Answer from the drawing. Dimensions are ordinates in mm from the lowest x, y and z of the part. A direction names the side the tool comes from. Give positions to 0.01 mm unless a question says otherwise; leave off trailing zeros. Loops run counter-clockwise (first coordinate to the right, second up) from the corner with the lowest first, then second, coordinate; pieces in that order, holes last. Notation, with made-up numbers: (-18, 21) -> (37, 21) arc R24 ccw to (37, 31) -> close; hole circle Ø3 at (-16.75, -31). An arc over 180 degrees is marked (long way). Return JSON: item names as keys, results as strings. Group by question number.
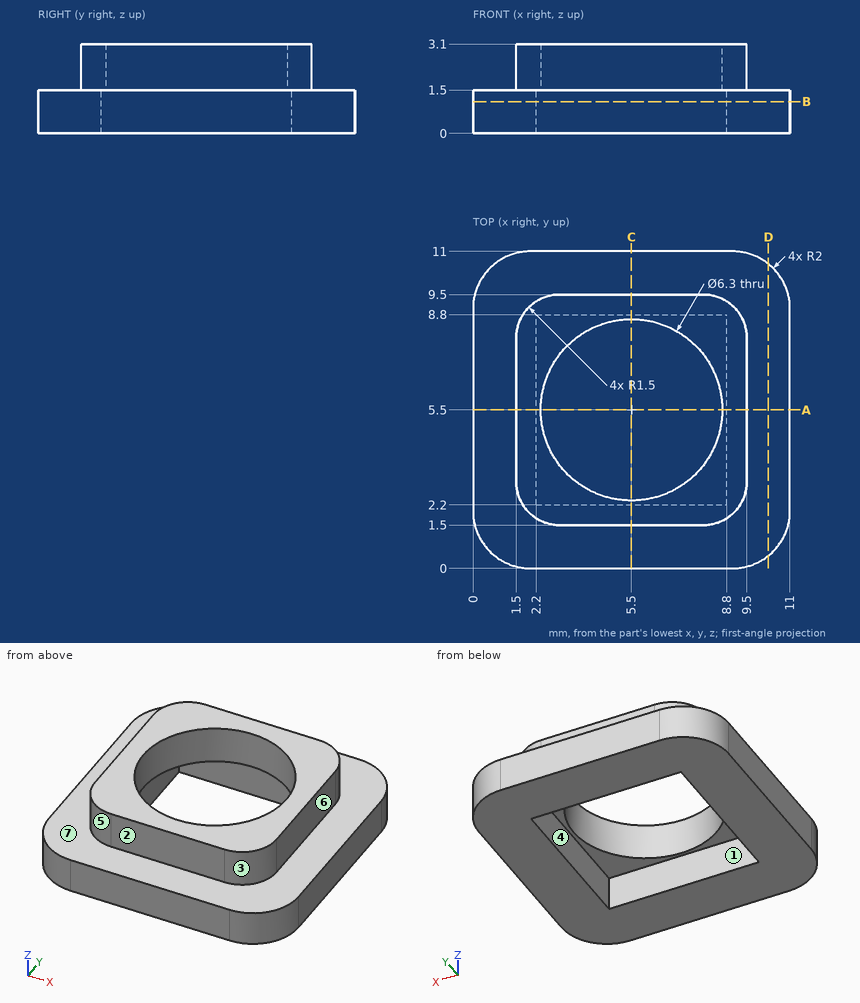
1. Straight lines are drawn through the part: line 1 (Y direction, x = 5.5, z = 2); line 2 (Y direction, x = 6, z = 1). For each, find the intervals that lie inside material, in ascending order. Write a range as from..to.
2. Section A-A on y = 5.5 is taken. Determine the outline of the cut face in (x, z).
3. Section D-D on x = 10.25 is taken. Determine the outline of the cut face in (y, z).
4. Section B-B on z = 1.1 is taken. Determine the outline of the cut face in (x, y), then the cut area to 3 significant figures.
5. Which of the six approach directions +Z, -Z, +X, -X, +Y, -Y give full straight-line access (tool end or side, diameter ignored) to the marked faces 4, 5, 6 and 7?
6. Flat-ended cylindrical pins translate along their axes: pin 1 Ø0.8 at (y, z) = (6, 2.5) entering from +X; pin 2 Ø1.3 at (y, z) = (5.5, 2.5) entering from -X; pin 3 Ø1.3 at (x, z) = (5.5, 2.5) entering from -Y. Find the tip coordinate at first contact, or state that the pin passes through.
7. Determine the mould class of the marked faces 1, 2 and 3 for opening direction X: pulls with the +X half, pulls with the -X half, needs draft (parallel to the pull), parting line crosses it, or undercut.
Completed:
{
 "1": {"line 1": "y = 1.5..2.35, 8.65..9.5", "line 2": "y = 0..2.2, 8.8..11"},
 "2": {"outline": "(0, 0) -> (2.2, 0) -> (2.2, 1.5) -> (2.35, 1.5) -> (2.35, 3.1) -> (1.5, 3.1) -> (1.5, 1.5) -> (0, 1.5) -> close; (8.65, 1.5) -> (8.8, 1.5) -> (8.8, 0) -> (11, 0) -> (11, 1.5) -> (9.5, 1.5) -> (9.5, 3.1) -> (8.65, 3.1) -> close"},
 "3": {"outline": "(0.44, 0) -> (10.56, 0) -> (10.56, 1.5) -> (0.44, 1.5) -> close"},
 "4": {"outline": "(0, 2) arc R2 ccw to (2, 0) -> (9, 0) arc R2 ccw to (11, 2) -> (11, 9) arc R2 ccw to (9, 11) -> (2, 11) arc R2 ccw to (0, 9) -> close; hole (2.2, 2.2) -> (8.8, 2.2) -> (8.8, 8.8) -> (2.2, 8.8) -> close", "area": "74.0 mm²"},
 "5": {"face 4": "-Z", "face 5": "+Z, -X, -Y", "face 6": "+Z, +X, +Y, -Y", "face 7": "+Z"},
 "6": {"pin 1": "stops at x = 9.5", "pin 2": "stops at x = 1.5", "pin 3": "stops at y = 1.5"},
 "7": {"face 1": "undercut", "face 2": "needs draft", "face 3": "pulls with the +X half"}
}
